Here's how the part is built. I have some questions about the finished solid (model axes, mm). A direction names the side the tool comes from. Round coordinates to 2 decimals unless told otherwise and drop trailing zeros. Loops run counter-clockwise (first coordinate to the right, second up) from the corner with the lowest first, then second, coordinate; pieces in that order, holes last. Notation, with made-up numbers: M 62,2 L 69,2 A22 ccw 69,19 Z; hole C 55,-12.5 d2. An arc over 180 degrees is marked long. Put each result on its own line as item: value. Start each with the question number.
```python
from build123d import *

# Parameters (mm, degrees)
F0_W     = 4
F0_H     = 4
F0_W_2   = 10
F0_H_2   = 8
F1_DEPTH = 35


with BuildPart() as f1:
    # F0 (on Top) → F1 (new body)
    with BuildSketch(Plane.XY):
        Polygon((-4, 31), (0, 31), (4, 37.928203), (0, 37.928203), align=None)
        Polygon((-4, 0), (0, 0), (0, 8), (0, 31), (-4, 31), align=None)
        with Locations((-2, -2)):
            Rectangle(F0_W, F0_H)
        Polygon((10, 0), (0, 0), (0, -4), (52, -4), (52, 0), (42, 0), align=None)
        with Locations((54, -2)):
            Rectangle(F0_W, F0_H)
        Polygon((52, 8), (52, 0), (56, 0), (56, 31), (52, 31), align=None)
        Polygon((48, 37.928203), (52, 31), (56, 31), (52, 37.928203), align=None)
        with Locations((5, 4)):
            Rectangle(F0_W_2, F0_H_2)
        with Locations((47, 4)):
            Rectangle(F0_W_2, F0_H_2)
    extrude(amount=F1_DEPTH)


solid = f1.part
```
1) Suppose I cut it at C-C (y = 29). Write out the boundary of the cut face in (x, z), plus the area to 3 significant figures.
2) If we mould it in two halves opening along Y, with no side actions, what happens to faces 1 (the face through (-1.972, 34.513, 17.255)), 2 (the face through (49.972, 34.513, 17.255)), 3 (the face through (10, 4, 17)), 4 (the face through (1.972, 34.416, 17.255))? For each: pulls with the +Y half, pulls with the -Y half, needs draft (parallel to the pull), parting line crosses it, or undercut.
3) Suppose I cut it at A-A (y = 1.5). Write out the boundary of the cut face in (x, z).
4) If I drill on probe 1 along X at (y, z) = (19.5, 26); probe 2 along X at (y, z) = (3.5, 31); probe 3 along Y at (x, z) = (18, 8.5), over which ranges is the centre line in solid material (lowest first)? Write a range as from..to.
5) Suppose I cut it at B-B (z = 18). Write out the boundary of the cut face in (x, y).
6) I'm going to push flat-ended pins straight in: P1, Ø3, axis at x = 7.5, z = 9.5, coming from the +Y side; P2, Ø10, axis at x = 35, z = 16, coming from the +Y side. Where does each tip first touch, or does it pass through?
7) On a 3-axis mill with a long thin cutter (end or side, diameter ignored), from which of +Z, -Z, +X, -X, +Y, -Y can I reach the whole of each face in a straight line? I mean faces 5 (the face through (28, -2, 0)), 6 (the face through (42, 4, 17)), 7 (the face through (52, 20, 17)). Say none if no direction works.
8) Suppose I cut it at D-D (x = 29). Write out the boundary of the cut face in (y, z), plus the area to 3 significant figures.
Results are:
1. outline: M -4,0 L 0,0 L 0,35 L -4,35 Z; M 52,0 L 56,0 L 56,35 L 52,35 Z
1. area: 280 mm²
2. face 1: pulls with the +Y half
2. face 2: undercut
2. face 3: needs draft
2. face 4: undercut
3. outline: M -4,0 L 10,0 L 10,35 L -4,35 Z; M 42,0 L 56,0 L 56,35 L 42,35 Z
4. probe 1: -4..0, 52..56
4. probe 2: -4..10, 42..56
4. probe 3: -4..0
5. outline: M -4,-4 L 56,-4 L 56,31 L 52,37.93 L 48,37.93 L 52,31 L 52,8 L 42,8 L 42,0 L 10,0 L 10,8 L 0,8 L 0,31 L 4,37.93 L 0,37.93 L -4,31 Z
6. P1: y = 8
6. P2: y = 0
7. face 5: -Z, +X, -X, +Y, -Y
7. face 6: +Z, -Z, +Y
7. face 7: +Z, -Z
8. outline: M -4,0 L 0,0 L 0,35 L -4,35 Z
8. area: 140 mm²
